```python
from build123d import *

# Parameters (mm, degrees)
SKETCH2_R           = 40
SKETCH2_R_2         = 2.75
BOSS_EXTRUDE1_DEPTH = 5
FILLET1_R           = 2
SKETCH3_R           = 12.5
SKETCH3_R_2         = 2.75
BOSS_EXTRUDE2_DEPTH = 3.69
SKETCH4_R           = 1
CUT_EXTRUDE1_DEPTH  = 58.23212479


with BuildPart() as part:
    # Sketch2 → Boss-Extrude1 (new body)
    with BuildSketch(Plane(origin=(0, 0, 0), x_dir=(1, 0, 0), z_dir=(0, 1, 0))):
        with Locations(Location((0, 0, 0), (0, 0, 270))):
            Circle(SKETCH2_R)
        with Locations(Location((0, 0, 0), (0, 0, 270))):
            Circle(SKETCH2_R_2, mode=Mode.SUBTRACT)
    extrude(amount=BOSS_EXTRUDE1_DEPTH)

    # Fillet1
    fillet1_edges = [part.edges().sort_by_distance(p)[0] for p in [
        (0, 5, -40),
    ]]
    fillet(fillet1_edges, radius=FILLET1_R)

    # Sketch3 → Boss-Extrude2 (add)
    with BuildSketch(Plane(origin=(0, 5, 0), x_dir=(1, 0, 0), z_dir=(0, 1, 0))):
        with Locations(Location((0, 0, 0), (0, 0, 270))):
            Circle(SKETCH3_R)
        with Locations(Location((0, 0, 0), (0, 0, 270))):
            Circle(SKETCH3_R_2, mode=Mode.SUBTRACT)
    extrude(amount=BOSS_EXTRUDE2_DEPTH)

    # Sketch4 → Cut-Extrude1 (cut, through all)
    with BuildSketch(Plane(origin=(0, 8.69, 0), x_dir=(1, 0, 0), z_dir=(0, 1, 0))):
        with Locations(Location((-8.25, -3.15, 0), (0, 0, 270))):
            Circle(SKETCH4_R)
        with Locations(Location((19.25, -2.65, 0), (0, 0, 270))):
            Circle(SKETCH4_R)
    extrude(amount=-CUT_EXTRUDE1_DEPTH, mode=Mode.SUBTRACT)


solid = part.part
```
The listing builds one solid part. Answer for the finished solid, in the listing's coordinates (mm). A direction names the side the tool comes from. Round coordinates to 2 decimals unless told otherwise and drop trailing zeros. Loops run counter-clockwise (first coordinate to the right, second up) from the corner with the lowest first, then second, coordinate; pieces in that order, holes last. Notation, with made-up numbers: (60.5, 60.25) -> (101.5, 60.25) arc R33 cw to (101.5, 96.25) -> close; hole circle Ø1 at (-4, 16.25). An arc over 180 degrees is marked (long way). Use one line per item in the form item = value.
1. For a pull along Z with two mould halves and no side action, classify faces 3 (the cylindrical face through (-39.05, 1.48, -8.67)), 4 (the cylindrical face through (-2.685, 4.284, -0.596)), 5 (the flat face through (9, 5, -9)) as released by +Z, released by -Z, zero draft, split by the parting line, or undercut.
Answer key:
face_3 = split by the parting line
face_4 = undercut
face_5 = zero draft
2. Flat-ended cylindrical pins translate along their axes: pin 1 Ø1.5 at (x, y) = (-14.5, 5) entering from +Z; pin 2 Ø8 at (x, z) = (-26.5, 5) entering from +Y; pin 3 Ø1.6 at (x, z) = (19.25, 2.65) entering from +Y; pin 4 Ø5 at (y, z) = (5.5, -25) entering from -X. Find the tip coordinate at first contact, or state that the pin passes through.
Answer key:
pin_1 = 36.87
pin_2 = 5
pin_3 = through
pin_4 = -32.41
3. Find the intervals of material crossed by probe 1 along X at (y, z) = (5.75, 0); probe 2 along X at (y, z) = (2.5, 0); probe 3 along X at (y, z) = (3, 2), in increasing order. Write a range as [from, to].
Answer key:
probe_1 = [-12.5, -2.75], [2.75, 12.5]
probe_2 = [-40, -2.75], [2.75, 40]
probe_3 = [-39.95, -1.89], [1.89, 18.49], [20.01, 39.95]
4. A tool of negligible diameter and unlimited length cuts with its end or side. For faces 1 (the cylindrical face through (18.36, 2.54, 3.11)), 2 (the cylindrical face through (3.755, 6.819, 11.923)), from which of +Z, -Z, +X, -X, +Y, -Y can it reach the whole face along a straight path? Write none if from no direction.
Answer key:
face_1 = +Y, -Y
face_2 = +Y
5. The part is cut by section B-B on x = 0. Determine the outline of the cut face in (y, z).
Answer key:
outline = (0, -40) -> (3, -40) arc R2 ccw to (5, -38) -> (5, -12.5) -> (8.69, -12.5) -> (8.69, -2.75) -> (0, -2.75) -> close; (0, 2.75) -> (8.69, 2.75) -> (8.69, 12.5) -> (5, 12.5) -> (5, 38) arc R2 ccw to (3, 40) -> (0, 40) -> close
6. The part is cut by section C-C on y = 1.5. Determine the outline of the cut face in (x, z), and give its area (3 significant figures).
Answer key:
outline = circle Ø80 at (0, 0); hole circle Ø2 at (-8.25, 3.15); hole circle Ø5.5 at (0, 0); hole circle Ø2 at (19.25, 2.65)
area = 5,000 mm²
7. The part is cut by section A-A on z = 0. Determine the outline of the cut face in (x, y), and give its area (3 significant figures).
Answer key:
outline = (-40, 0) -> (-2.75, 0) -> (-2.75, 8.69) -> (-12.5, 8.69) -> (-12.5, 5) -> (-38, 5) arc R2 ccw to (-40, 3) -> close; (2.75, 0) -> (40, 0) -> (40, 3) arc R2 ccw to (38, 5) -> (12.5, 5) -> (12.5, 8.69) -> (2.75, 8.69) -> close
area = 443 mm²
